Build history of the part. All positions in model axes, mm. Give positions to 0.01 mm unless a question says otherwise; leave off trailing zeros. Write each loop counter-clockwise with the first axis right and the second up, starting at its lowest first coordinate (ties: lowest second). Pieces come first, ordered by that corner, then holes. Notation, with made-up numbers: (75.5, 0) -> (89.5, 0) arc R24 cw to (89.5, 19) -> close; hole circle Ø9 at (30.25, 25). An arc over 180 degrees is marked (long way). Put each result on its own line as item: value.
from build123d import *

# Parameters (mm, degrees)
SKETCH1_W           = 48
SKETCH1_H           = 36
SKETCH1_R           = 2
BOSS_EXTRUDE1_DEPTH = 2
SKETCH2_W           = 140
SKETCH2_H           = 80
BOSS_EXTRUDE2_DEPTH = 3


with BuildPart() as part:
    # Sketch1 → Boss-Extrude1 (new body)
    with BuildSketch(Plane.XY):
        Rectangle(SKETCH1_W, SKETCH1_H)
        with Locations((-19, 11)):
            Circle(SKETCH1_R, mode=Mode.SUBTRACT)
        with Locations((-19, -13)):
            Circle(SKETCH1_R, mode=Mode.SUBTRACT)
        with Locations((19, -13)):
            Circle(SKETCH1_R, mode=Mode.SUBTRACT)
        with Locations((19, 11)):
            Circle(SKETCH1_R, mode=Mode.SUBTRACT)
    extrude(amount=BOSS_EXTRUDE1_DEPTH)

    # Sketch2 → Boss-Extrude2 (add)
    with BuildSketch(Plane(origin=(0, 18, 0), x_dir=(1, 0, 0), z_dir=(0, 1, 0))):
        with Locations((4, 38)):
            Rectangle(SKETCH2_W, SKETCH2_H)
    extrude(amount=BOSS_EXTRUDE2_DEPTH)


solid = part.part
1) Slice it at D-D (z = -8). Write the cut outline in (x, y).
Filled sheet:
outline: (-66, 18) -> (74, 18) -> (74, 21) -> (-66, 21) -> close
2) Slice it at C-C (y = 16.5). Write the cut outline in (x, z).
Filled sheet:
outline: (-24, 0) -> (24, 0) -> (24, 2) -> (-24, 2) -> close
3) Wall check: L1, parallel to Y at x = -19, z = 0.7; L2, parallel to Z at x = -5.5, y = 5.5; L3, parallel to Y at x = 61, z = -52.5. Give the ranges that are in metal, low to high.
Filled sheet:
L1: -18 to -15, -11 to 9, 13 to 21
L2: 0 to 2
L3: 18 to 21
4) Pull direction X, two halves, no side cores. Call faces 1 (the cylindrical face through (-20.474, -11.648, 0.986)), 2 (the flat face through (-66, 19, -37)), 3 (the flat face through (0, 0, 0)): released by +X, released by -X, zero draft, split by the parting line, or undercut.
Filled sheet:
face 1: undercut
face 2: released by -X
face 3: zero draft
5) Pin check, flat tips, straight feed: pin 1 (6.5 mm diameter, centred on x = 19, y = 11, fed in from -Z); pin 2 (8 mm diameter, centred on x = -22.5, z = -52.5, fed in from -Y); pin 3 (0.6 mm diameter, centred on y = -2, z = 1, fed in from +X); pin 4 (3.5 mm diameter, centred on x = -19, y = 11, fed in from -Z). Stop position of each tip, or through.
Filled sheet:
pin 1: z = 0
pin 2: y = 18
pin 3: x = 24
pin 4: through
6) Slice it at A-A (x = 19). Write the cut outline in (y, z), plus the area to 3 significant figures.
Filled sheet:
outline: (-18, 0) -> (-15, 0) -> (-15, 2) -> (-18, 2) -> close; (-11, 0) -> (9, 0) -> (9, 2) -> (-11, 2) -> close; (13, 0) -> (18, 0) -> (18, -78) -> (21, -78) -> (21, 2) -> (13, 2) -> close
area: 296 mm2
7) Slice it at B-B (y = -13). Write the cut outline in (x, z), plus the area to 3 significant figures.
Filled sheet:
outline: (-24, 0) -> (-21, 0) -> (-21, 2) -> (-24, 2) -> close; (-17, 0) -> (17, 0) -> (17, 2) -> (-17, 2) -> close; (21, 0) -> (24, 0) -> (24, 2) -> (21, 2) -> close
area: 80.0 mm2
